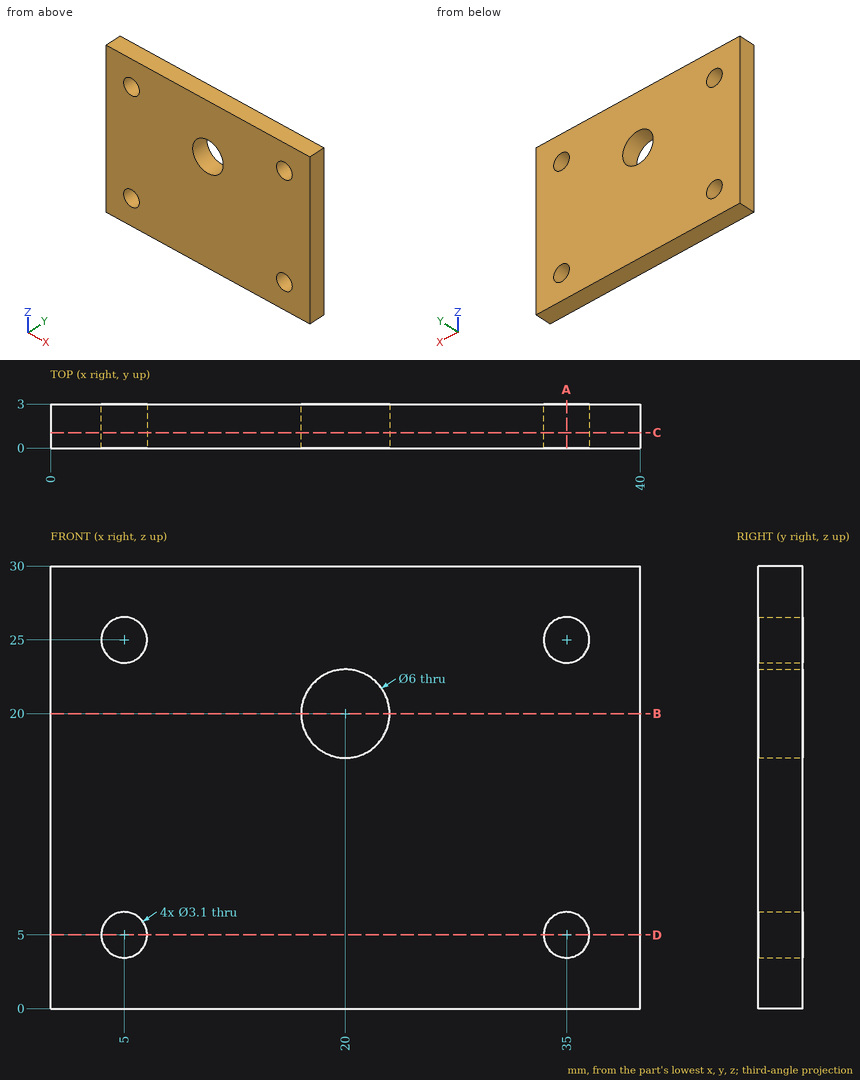
Answer from the drawing. Dimensions are ordinates in mm from the lowest x, y and z of the part. Coordinates: 2 decimals unless noted, no trailing zeros. Order: outer loops, then holes, each group sorted by start corner. A loop starts at its lowest first (then second) coordinate and runs counter-clockwise, first axis right, second up. Notation, with made-up numbers: (-8, 69.25) -> (24, 69.25) arc R29 ccw to (24, 107.25) -> close; hole circle Ø2 at (45.25, -20.5). An arc over 180 degrees is marked (long way). Answer as a JSON object with one key per item and string values.
1) A cutting plane is placed at A-A, the plane x = 35. Determine the outline of the cut face in (y, z), plus the area to 3 significant figures.
Model answer:
{"outline": "(0, 0) -> (3, 0) -> (3, 3.45) -> (0, 3.45) -> close; (0, 6.55) -> (3, 6.55) -> (3, 23.45) -> (0, 23.45) -> close; (0, 26.55) -> (3, 26.55) -> (3, 30) -> (0, 30) -> close", "area": "71.4 mm²"}
2) A cutting plane is placed at B-B, the plane z = 20. Determine the outline of the cut face in (x, y), plus the area to 3 significant figures.
Model answer:
{"outline": "(0, 0) -> (17, 0) -> (17, 3) -> (0, 3) -> close; (23, 0) -> (40, 0) -> (40, 3) -> (23, 3) -> close", "area": "102 mm²"}
3) This flat-tipped pin is pushed along its axis until it touches: pin 1 (3 mm diameter, centred on x = 5, z = 25, fed in from +Y). Where does it stop, or does it pass through?
Model answer:
{"pin 1": "passes through"}
4) A cutting plane is placed at C-C, the plane y = 1.05. Determine the outline of the cut face in (x, z).
Model answer:
{"outline": "(0, 0) -> (40, 0) -> (40, 30) -> (0, 30) -> close; hole circle Ø3.1 at (5, 5); hole circle Ø3.1 at (5, 25); hole circle Ø6 at (20, 20); hole circle Ø3.1 at (35, 5); hole circle Ø3.1 at (35, 25)"}
5) Consider line 1 along Z through (x, y) = (5, 1.6); line 2 along X through (y, z) = (0.4, 5.75); line 3 along Z through (x, y) = (20, 2.75). Determine where each line is inside the solid, lowest interval first. Write a range as from..to.
Model answer:
{"line 1": "z = 0..3.45, 6.55..23.45, 26.55..30", "line 2": "x = 0..3.64, 6.36..33.64, 36.36..40", "line 3": "z = 0..17, 23..30"}
6) A cutting plane is placed at D-D, the plane z = 5. Determine the outline of the cut face in (x, y), plus the area to 3 significant figures.
Model answer:
{"outline": "(0, 0) -> (3.45, 0) -> (3.45, 3) -> (0, 3) -> close; (6.55, 0) -> (33.45, 0) -> (33.45, 3) -> (6.55, 3) -> close; (36.55, 0) -> (40, 0) -> (40, 3) -> (36.55, 3) -> close", "area": "101 mm²"}
